from build123d import *

# Parameters (mm, degrees)
SKETCH1_W           = 559
SKETCH1_H           = 762
BOSS_EXTRUDE1_DEPTH = 1.6
SKETCH2_W           = 559
SKETCH2_H           = 762
SKETCH2_W_2         = 555.8
SKETCH2_H_2         = 758.8
BOSS_EXTRUDE2_DEPTH = 25
SKETCH3_R           = 6.35
CUT_EXTRUDE1_DEPTH  = 2.6


with BuildPart() as part:
    # Sketch1 → Boss-Extrude1 (new body)
    with BuildSketch(Plane(origin=(0, 0, 0), x_dir=(1, 0, 0), z_dir=(0, 1, 0))):
        with Locations((279.5, 381)):
            Rectangle(SKETCH1_W, SKETCH1_H)
    extrude(amount=BOSS_EXTRUDE1_DEPTH)

    # Sketch2 → Boss-Extrude2 (add)
    with BuildSketch(Plane(origin=(0, 1.6, 0), x_dir=(1, 0, 0), z_dir=(0, 1, 0))):
        with Locations((279.5, 381)):
            Rectangle(SKETCH2_W, SKETCH2_H)
        with Locations((279.5, 381)):
            Rectangle(SKETCH2_W_2, SKETCH2_H_2, mode=Mode.SUBTRACT)
    extrude(amount=BOSS_EXTRUDE2_DEPTH)

    # Sketch3 → Cut-Extrude1 (cut, through all)
    with BuildSketch(Plane(origin=(0, 1.6, 0), x_dir=(1, 0, 0), z_dir=(0, 1, 0))):
        with Locations((532.4, 735.4)):
            Circle(SKETCH3_R)
    extrude(amount=-CUT_EXTRUDE1_DEPTH, mode=Mode.SUBTRACT)


solid = part.part
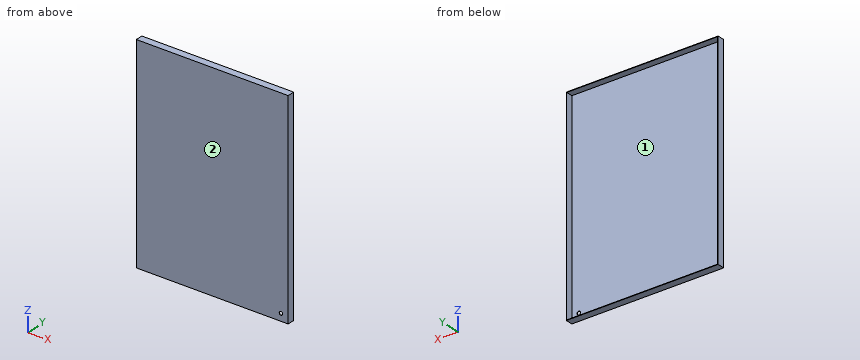
Verification items for the finished model (mm, model axes). Face numbers are marked on the shaded views. Coordinates: 2 decimals unless noted, no trailing zeros. Order: outer loops, then holes, each group sorted by start corner. A loop starts at its lowest first (then second) coordinate and runs counter-clockwise, first axis right, second up. Notation, with made-up numbers: M -28.5,61 L -9.5,61 A19 cw -9.5,85 Z; hole C 72,83 d4. An arc over 180 degrees is marked long. One line per item, written item: value. Start each with the question number.
Item 1: Scan lines: probe 1 along X at (y, z) = (11, -525.5); probe 2 along Z at (x, y) = (193, 7); probe 3 along X at (y, z) = (0.4, -735.4). Record each from-to range of solid material in increasing order.
Item 2: Sectioned sample at B-B (x = 236). Enter the section's corners in (y, z), then the cut area to 3 significant figures.
Item 3: Sectioned sample at C-C (z = -55.5). Enter the section's corners in (x, y), then the cut area to 3 significant figures.
Item 4: Mould release check, pull along Z, two halves, no side actions. Record for the marked faces 1 and 2: released by +Z, released by -Z, zero draft, split by the parting line, or undercut.
Item 5: Sectioned sample at A-A (y = 16.5). Enter the section's corners in (x, z).
Item 6: Gauge pin test, flat ends, axial feed: pin 1 (1.5 mm diameter, centred on x = 164, z = -141, fed in from +Y); pin 2 (7.5 mm diameter, centred on x = 360, y = 17, fed in from +Z). Record the tip position at first contact, or that the pin passes through.
Conclusion:
1. probe 1: x = 0 to 1.6, 557.4 to 559
1. probe 2: z = -762 to -760.4, -1.6 to 0
1. probe 3: x = 0 to 526.05, 538.75 to 559
2. outline: M 0,-762 L 26.6,-762 L 26.6,-760.4 L 1.6,-760.4 L 1.6,-1.6 L 26.6,-1.6 L 26.6,0 L 0,0 Z
2. area: 1,300 mm^2
3. outline: M 0,0 L 559,0 L 559,26.6 L 557.4,26.6 L 557.4,1.6 L 1.6,1.6 L 1.6,26.6 L 0,26.6 Z
3. area: 974 mm^2
4. face 1: undercut
4. face 2: zero draft
5. outline: M 0,-762 L 559,-762 L 559,0 L 0,0 Z; hole M 1.6,-760.4 L 557.4,-760.4 L 557.4,-1.6 L 1.6,-1.6 Z
6. pin 1: stops at y = 1.6
6. pin 2: stops at z = 0
